from build123d import *

# Parameters (mm, degrees)
F1_DEPTH = 44
F0_W     = 114
F0_H     = 50
F0_R     = 11.1
F2_DEPTH = 22
F3_DEPTH = 64
F4_DEPTH = 74
F5_SIZE2 = 12
F5_SIZE  = 12


with BuildPart() as f1:
    # F0 (on Front) → F1 (new body)
    with BuildSketch(Plane.XZ):
        with BuildLine():
            ThreePointArc((35.142567, 41), (45.124741, 29.660711), (51.575188, 16))
            ThreePointArc((51.575188, 16), (53.390356, 8.091349), (54, 0))
            ThreePointArc((54, 0), (53.390356, -8.091349), (51.575188, -16))
            ThreePointArc((51.575188, -16), (45.124741, -29.660711), (35.142567, -41))
            Line((35.142567, -41), (174, -41))
            Line((174, -41), (174, -25))
            Line((174, -25), (60, -25))
            Line((60, -25), (60, 25))
            Line((60, 25), (174, 25))
            Line((174, 25), (174, 41))
            Line((174, 41), (35.142567, 41))
        make_face()
    extrude(amount=F1_DEPTH)

    # F0 (on Front) → F2 (join)
    with BuildSketch(Plane.XZ):
        with Locations((117, 0)):
            Rectangle(F0_W, F0_H)
        with Locations((84, 0)):
            Circle(F0_R, mode=Mode.SUBTRACT)
        with Locations((139, 0)):
            Circle(F0_R, mode=Mode.SUBTRACT)
    extrude(amount=F2_DEPTH)

    # F0 (on Front) → F3 (join)
    with BuildSketch(Plane.XZ):
        with BuildLine():
            ThreePointArc((-23.675528, 16), (0, 28.575), (23.675528, 16))
            Line((23.675528, 16), (51.575188, 16))
            ThreePointArc((51.575188, 16), (45.124741, 29.660711), (35.142567, 41))
            ThreePointArc((35.142567, 41), (-14.958535, 51.886821), (-51.575188, 16))
            Line((-51.575188, 16), (-23.675528, 16))
        make_face()
        with BuildLine():
            Line((51.575188, -16), (23.675528, -16))
            ThreePointArc((23.675528, -16), (0, -28.575), (-23.675528, -16))
            Line((-23.675528, -16), (-51.575188, -16))
            ThreePointArc((-51.575188, -16), (-14.958535, -51.886821), (35.142567, -41))
            ThreePointArc((35.142567, -41), (45.124741, -29.660711), (51.575188, -16))
        make_face()
    extrude(amount=F3_DEPTH)

    # F0 (on Front) → F4 (join)
    with BuildSketch(Plane.XZ):
        with BuildLine():
            ThreePointArc((23.675528, 16), (27.322691, 8.366672), (28.575, 0))
            ThreePointArc((28.575, 0), (27.322691, -8.366672), (23.675528, -16))
            Line((23.675528, -16), (51.575188, -16))
            ThreePointArc((51.575188, -16), (53.390356, -8.091349), (54, 0))
            ThreePointArc((54, 0), (53.390356, 8.091349), (51.575188, 16))
            Line((51.575188, 16), (23.675528, 16))
        make_face()
        with BuildLine():
            ThreePointArc((-23.675528, -16), (-28.575, 0), (-23.675528, 16))
            Line((-23.675528, 16), (-51.575188, 16))
            ThreePointArc((-51.575188, 16), (-54, 0), (-51.575188, -16))
            Line((-51.575188, -16), (-23.675528, -16))
        make_face()
    extrude(amount=F4_DEPTH)

    # F5
    f5_edges = [f1.edges().sort_by_distance(p)[0] for p in [
        (174, -44, -33),
        (174, -44, 33),
    ]]
    chamfer(f5_edges, length=F5_SIZE, length2=F5_SIZE2)


solid = f1.part
The listing builds one solid part. Answer for the finished solid, in the listing's coordinates (mm). A direction names the side the tool comes from. Give positions to 0.01 mm unless a question says otherwise; leave off trailing zeros. Write each loop counter-clockwise with the first axis right and the second up, starting at its lowest first coordinate (ties: lowest second). Pieces come first, ordered by that corner, then holes. Notation, with made-up numbers: (58, 68) - (70, 68) arc R21 ccw to (70, 101) - close; hole circle Ø11 at (55, -39). An arc over 180 degrees is marked (long way). Use a Markdown table: item, result.
1. Find the intervals of material crossed by probe 1 along Z at (x, y) = (84, -13); probe 2 along Z at (x, y) = (121, -36); probe 3 along Y at (x, z) = (67, -14), in increasing order. Write a range as from..to.
Values follow:
| item | result |
|---|---|
| probe 1 | z = -41..-11.1, 11.1..41 |
| probe 2 | z = -41..-25, 25..41 |
| probe 3 | y = -22..0 |
2. Section A-A on x = 139 is taken. Write down the section's boundary in (y, z).
Values follow:
| item | result |
|---|---|
| outline | (-44, -41) - (0, -41) - (0, -11.1) - (-22, -11.1) - (-22, -25) - (-44, -25) - close; (-44, 25) - (-22, 25) - (-22, 11.1) - (0, 11.1) - (0, 41) - (-44, 41) - close |
3. Section B-B on y = -38 is taken. Write down the section's boundary in (x, z) (3 decimals).
Values follow:
| item | result |
|---|---|
| outline | (-51.575, -16) arc R54 ccw to (35.143, -41) - (168, -41) - (168, -25) - (60, -25) - (60, 25) - (168, 25) - (168, 41) - (35.143, 41) arc R54 ccw to (-51.575, 16) arc R54 ccw to start; hole (23.676, -16) arc R28.575 ccw to (28.575, 0) arc R28.575 ccw to (23.676, 16) arc R28.575 ccw (long way) to start |
4. Section D-D on z = 19.5 is taken. Write down the section's boundary in (x, y), plus the area to 3 significant figures.
Values follow:
| item | result |
|---|---|
| outline | (-50.36, -64) - (-20.89, -64) - (-20.89, 0) - (-50.36, 0) - close; (20.89, -64) - (50.36, -64) - (50.36, -44) - (60, -44) - (60, -22) - (174, -22) - (174, 0) - (20.89, 0) - close |
| area | 6,700 mm² |
5. For a pull along X with two mould halves and no side action, classify faces 4 (the flat face through (60, -33, 0)), 5 (the flat face through (116, -33, 25)), 6 (the cylindrical face through (127.91, -10.85, 0.49)) as released by +X, released by -X, zero draft, split by the parting line, or undercut.
Values follow:
| item | result |
|---|---|
| face 4 | released by +X |
| face 5 | zero draft |
| face 6 | undercut |
6. Each of these flat-tipped pins is pushed along its axis until it touches: P1, Ø1, axis at x = -18, y = -61.5, coming from the +Z side; P2, Ø3, axis at y = -14.5, z = -5, coming from the -X side; P3, Ø8, axis at x = -14.5, y = -59.5, coming from the -Z side. Where does it stop, or does it pass through?
Values follow:
| item | result |
|---|---|
| P1 | stops at z = 51.09 |
| P2 | stops at x = -53.89 |
| P3 | stops at z = -52.97 |
7. Section C-C on y = -15.5 is taken. Write down the section's boundary in (x, z) (3 decimals), plus the area to 3 significant figures.
Values follow:
| item | result |
|---|---|
| outline | (-51.575, -16) arc R54 ccw to (35.143, -41) - (174, -41) - (174, 41) - (35.143, 41) arc R54 ccw to (-51.575, 16) arc R54 ccw to start; hole (23.676, -16) arc R28.575 ccw to (28.575, 0) arc R28.575 ccw to (23.676, 16) arc R28.575 ccw (long way) to start; hole circle Ø22.2 at (84, 0); hole circle Ø22.2 at (139, 0) |
| area | 16,100 mm² |
8. A tool of negligible diameter and unlimited length cuts with its end or side. For faces 1 (the flat face through (104, -22, -41)), 2 (the flat face through (-1, -64, 35)), 3 (the flat face through (118, -33, -25)), from which of +Z, -Z, +X, -X, +Y, -Y can it reach the whole face along a straight path? Write none if from no direction.
Values follow:
| item | result |
|---|---|
| face 1 | -Z, +X, +Y, -Y |
| face 2 | +Z, +X, -X, -Y |
| face 3 | +X, -Y |
